Drawing for the job (mm, zero at the part's lowest x, y, z). Give positions to 0.01 mm unless a question says otherwise; leave off trailing zeros. One line per item, written item: value.
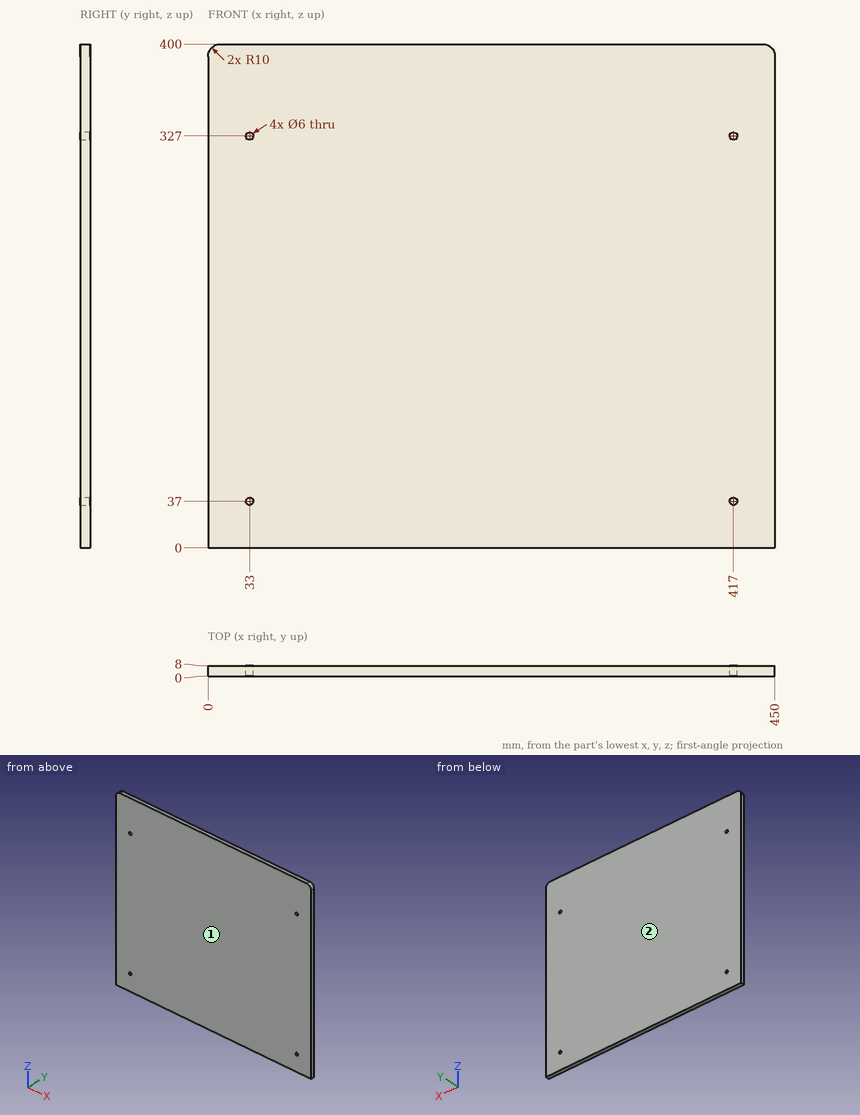
1) Mould opens along Y. For the marked faces 1 and 2 say: released by +Y, released by -Y, zero draft, split by the parting line, or undercut.
Check values:
face 1: released by -Y
face 2: released by +Y
2) Pin check, flat tip, straight feed: pin 1 (3 mm diameter, centred on x = 389.5, y = 2, fed in from -Z). Stop position of the tip, or through.
Check values:
pin 1: z = 0
3) Drill centre lines: probe 1 along X at (y, z) = (3.5, 37); probe 2 along Z at (x, y) = (417, 3.25). Where is each one in solid material? Low to high. Write a range as from..to.
Check values:
probe 1: 0..30, 36..414, 420..450
probe 2: 0..34, 40..324, 330..400
